Can you work these out from the drawing? Everything is in mm from the part's minimum corner. A direction names the side the tool comes from. Round coordinates to 2 decimals unless told otherwise and drop trailing zeros. Write each loop counter-clockwise with the first axis right and the second up, starting at its lowest first coordinate (ties: lowest second). Pieces come first, ordered by that corner, then holes.
Q1. If we section it at A-A (x = 9.5): Please give me the cut outline in (y, z).
Q2. If we section it at C-C (y = 11): Please give me the cut outline in (x, z).
Q3. I'm going to push flat-ended pins straight in: pin 1 Ø4.5 at (y, z) = (12, 12.5) entering from +X; pin 2 Ø3 at (y, z) = (11.5, 13) entering from -X; pin 3 Ø8 at (x, y) = (7, 2) entering from -Z. Where does each tip first touch, or does it pass through?
Q4. We'd pull the mould along X, two halves only. Please class the marked faces 1, 2, 3 and 4: +X half, -X half, draft (parallel to the pull), parting line (faces both ways), or undercut.
Q5. For the marked faces 5, 6, 7, 8 and 9, which set-ups out of +Z, -Z, +X, -X, +Y, -Y let a thin tool reach every point of the face, with its end or its side?
Q6. Please list where these lines run through material, in increasing order: line 1 along Z through (x, y) = (12, 1.75); line 2 along Y through (x, z) = (1.5, 5.25); line 3 along Z through (x, y) = (17.5, 19.5).
Q7. If we section it at D-D (x = 15.5): Please give me the cut outline in (y, z).
Q8. If we section it at B-B (z = 12.5): Please give me the cut outline in (x, y), plus the area to 3 significant figures.
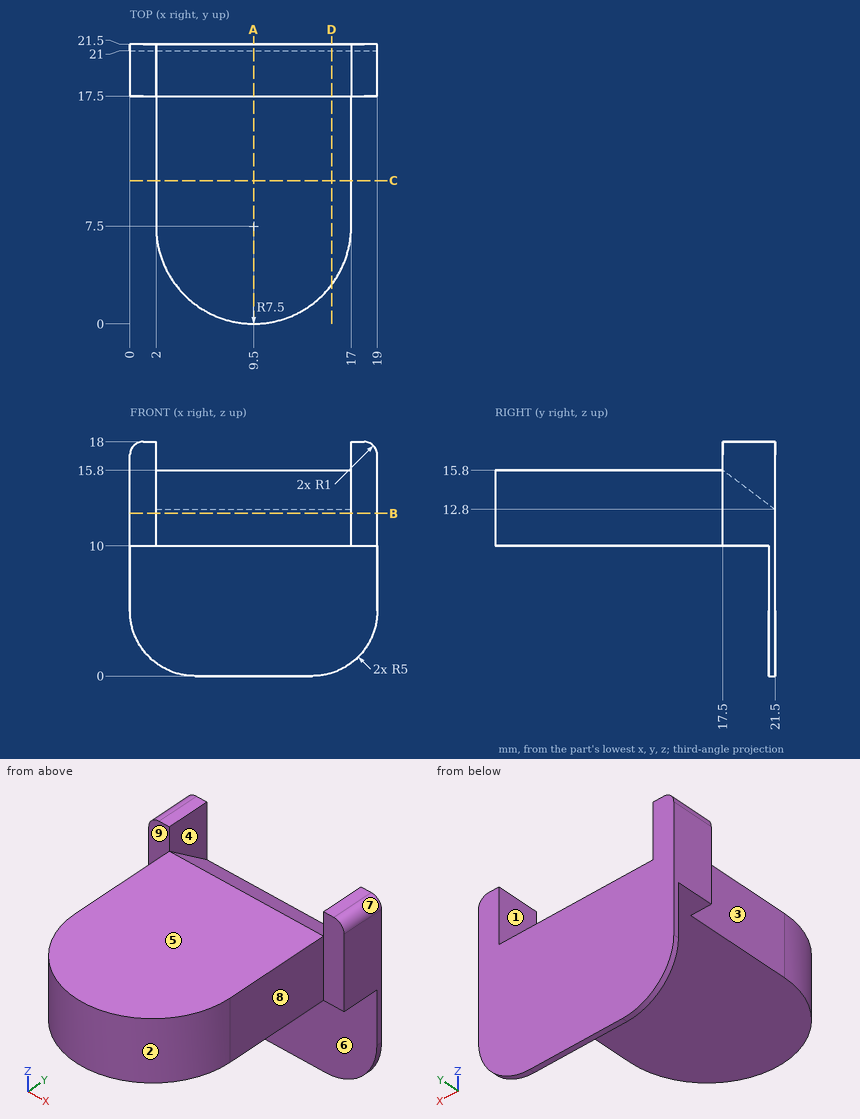
A:
1. outline: (0, 10) - (21, 10) - (21, 0) - (21.5, 0) - (21.5, 12.8) - (17.5, 15.8) - (0, 15.8) - close
2. outline: (2, 10) - (17, 10) - (17, 15.8) - (2, 15.8) - close
3. pin 1: stops at x = 17
3. pin 2: stops at x = 2
3. pin 3: stops at z = 10
4. face 1: undercut
4. face 2: parting line
4. face 3: -X half
4. face 4: undercut
5. face 5: +Z, +X, -X, +Y, -Y
5. face 6: -Z, +X, -X, -Y
5. face 7: +Z, +X, +Y, -Y
5. face 8: +Z, -Z, +X, -Y
5. face 9: +Z, -Z, -X, -Y
6. line 1: z = 10 to 15.8
6. line 2: y = 21 to 21.5
6. line 3: z = 10 to 18
7. outline: (3, 10) - (21, 10) - (21, 0.23) - (21.5, 0.23) - (21.5, 12.8) - (17.5, 15.8) - (3, 15.8) - close
8. outline: (0, 17.5) - (2, 17.5) - (2, 7.5) arc R7.5 ccw to (17, 7.5) - (17, 17.5) - (19, 17.5) - (19, 21.5) - (0, 21.5) - close
8. area: 314 mm2
